Can you work these out from the model? Positions are in its coordinate system, mm. Round coordinates to 2 decimals unless told otherwise and drop trailing zeros. Loops run counter-clockwise (first coordinate to the right, second up) from the corner with the lowest first, then second, coordinate; pieces in that order, holes last.
(1) I want a section at B-B on x = 0. Write out the boundary of the cut face in (y, z).
(2) If I drill on line 1 along X through (y, z) = (13.5, 0); line 2 along Y through (x, z) = (0, 22.8); line 3 along X through (y, z) = (18, -21.9), over which ranges is the centre line in solid material (lowest first)?
(3) Thinking about a two-plate mould opening in Z: for faces 1 (the face through (0, 20, -22)), 2 (the face through (-6.31, 17.76, -20.03)), 3 (the face through (9.19, 18.25, -22.17)), which applies, released by +Z, released by -Z, zero draft, split by the parting line, or undercut?
(4) I want a section at A-A on z = 0. Write out the boundary of the cut face in (x, y), plus the area to 3 significant figures.
(5) Will these pins go through, and if not, where does the flat tip stop? pin 1 Ø4 at (x, z) = (-6, 16.5) entering from -Y; pin 2 Ø3 at (x, y) = (-10.5, 20) entering from -Z; pin 3 Ø1 at (x, y) = (14.5, 24.5) entering from +Z; pin 4 Ø10 at (y, z) = (23, -12) entering from -X.
from build123d import *

# Parameters (mm, degrees)
ESQUISSE2_R                  = 2
ENL_V_MAT_EXTRU_1_DEPTH      = 25
ENL_V_MAT_EXTRU_1_DEPTH_BACK = 25


with BuildPart() as part:
    # Esquisse1 → Révolution1 (revolve)
    with BuildSketch(Plane.XY, mode=Mode.PRIVATE) as r_volution1_sk:
        Polygon((-24, 36), (-21.267949192, 36), (-21, 35), (-21, 1), (-21.267949192, 0), (-24, 0), align=None)
    revolve(r_volution1_sk.sketch.rotate(Axis((0, 0, 0), (0, 1, 0)), 270), axis=Axis((0, 0, 0), (0, 1, 0)))  # turned: the seam where the file's is

    # Esquisse2 → Enlèv. mat.-Extru.1 (cut, two sides)
    with BuildSketch(Plane.XY) as enl_v_mat_extru_1_sk:
        with Locations((0, 18)):
            Circle(ESQUISSE2_R)
    extrude(amount=ENL_V_MAT_EXTRU_1_DEPTH, mode=Mode.SUBTRACT)
    extrude(enl_v_mat_extru_1_sk.sketch, amount=-ENL_V_MAT_EXTRU_1_DEPTH_BACK, mode=Mode.SUBTRACT)


solid = part.part
Filled sheet:
1. outline: (0, -24) - (16, -24) - (16, -21) - (1, -21) - (0, -21.27) - close; (0, 21.27) - (1, 21) - (16, 21) - (16, 24) - (0, 24) - close; (20, -24) - (36, -24) - (36, -21.27) - (35, -21) - (20, -21) - close; (20, 21) - (35, 21) - (36, 21.27) - (36, 24) - (20, 24) - close
2. line 1: x = -24 to -21, 21 to 24
2. line 2: y = 0 to 16, 20 to 36
2. line 3: x = -9.82 to -2, 2 to 9.82
3. face 1: zero draft
3. face 2: undercut
3. face 3: split by the parting line
4. outline: (-24, 0) - (-21.27, 0) - (-21, 1) - (-21, 35) - (-21.27, 36) - (-24, 36) - close; (21, 1) - (21.27, 0) - (24, 0) - (24, 36) - (21.27, 36) - (21, 35) - close
4. area: 215 mm2
5. pin 1: passes through
5. pin 2: stops at z = -22.25
5. pin 3: stops at z = 19.49
5. pin 4: stops at x = -22.96
